Could you check a few things on this model? Use its own coordinates, in mm. A direction names the side the tool comes from. Coordinates: 2 decimals unless noted, no trailing zeros. Loops run counter-clockwise (first coordinate to the right, second up) from the corner with the lowest first, then second, coordinate; pieces in that order, holes last.
from build123d import *

# Parameters (mm, degrees)
BOSS_EXTRUDE1_DEPTH     = 18
CUT_EXTRUDE1_REACH      = 86.238
CUT_EXTRUDE1_END_RADIUS = 15
SKETCH3_R               = 7


with BuildPart() as part:
    # Sketch2 → Boss-Extrude1 (new body)
    with BuildSketch(Plane.XY):
        with BuildLine():
            Line((-33.38706816, 74), (-36, 74))
            Line((-36, 74), (-36, 0))
            Line((-36, 0), (-33, 0))
            Line((-33, 0), (-33, 35))
            ThreePointArc((-33, 35), (-18, 50), (-3, 35))
            Line((-3, 35), (-3, 0))
            Line((-3, 0), (0, 0))
            Line((0, 0), (0, 74))
            Line((0, 74), (-12.61679677, 74))
            Line((-12.61679677, 74), (-33.38706816, 74))
        make_face()
    extrude(amount=BOSS_EXTRUDE1_DEPTH)

    # Cut-Extrude1: up to this cylinder (the profile starts outside it)
    cut_extrude1_end = Plane(origin=(-18, 35, 9), z_dir=(0, 0, -1)) * Cylinder(CUT_EXTRUDE1_END_RADIUS, 203.476, mode=Mode.PRIVATE)
    # Sketch3 → Cut-Extrude1 (cut, up to the surface)
    with BuildSketch(Plane(origin=(0, 74, 0), x_dir=(1, 0, 0), z_dir=(0, 1, 0)), mode=Mode.PRIVATE) as cut_extrude1_sk1:
        with Locations(Location((-18, -9, 0), (0, 0, 270))):
            Circle(SKETCH3_R)
    cut_extrude1_tool1 = extrude(cut_extrude1_sk1.sketch, amount=-CUT_EXTRUDE1_REACH, mode=Mode.PRIVATE) - cut_extrude1_end
    add(cut_extrude1_tool1.solids().sort_by_distance((-18, 74, 9))[0], mode=Mode.SUBTRACT)


solid = part.part
(1) Imagine slicing it at D-D, the plane y = 67. Write out the boundary of the cut face in (x, z), and give its area (3 significant figures).
Answers:
outline: (-36, 0) - (0, 0) - (0, 18) - (-36, 18) - close; hole circle Ø14 at (-18, 9)
area: 494 mm2
(2) Imagine slicing it at A-A, the plane y = 8. Write out the boundary of the cut face in (x, z), and give its area (3 significant figures).
Answers:
outline: (-36, 0) - (-33, 0) - (-33, 18) - (-36, 18) - close; (-3, 0) - (0, 0) - (0, 18) - (-3, 18) - close
area: 108 mm2
(3) Which directions (+Z, -Z, +X, -X, +Y, -Y) give clear straight access to the entire face, cutting with the end or side of a thin tool? Please do faces 1 (the face through (-2, 0, 9)), 2 (the face through (-33, 17, 9)).
Answers:
face 1: +Z, -Z, +X, -X, -Y
face 2: +Z, -Z, -Y
(4) Imagine slicing it at B-B, the plane x = -18. Write out the boundary of the cut face in (y, z), and give its area (3 significant figures).
Answers:
outline: (50, 0) - (74, 0) - (74, 2) - (50, 2) - close; (50, 16) - (74, 16) - (74, 18) - (50, 18) - close
area: 96.0 mm2
(5) For pin 1 (6 mm diameter, centred on x = -4, z = 2.5, fed in from -Y); pin 2 (1.5 mm diameter, centred on x = -9.5, z = 2.5, fed in from -Y); pin 3 (8 mm diameter, centred on x = -10.5, y = 39.5, fed in from +Z), each with a flat end and sliding along its axis, tell me the tip position at first contact or that it passes through.
Answers:
pin 1: stops at y = 0
pin 2: stops at y = 46.81
pin 3: passes through
(6) We'd pull the mould along X, two halves only. Please class faces 3 (the face through (0, 36, 9)), 4 (the face through (-3, 18, 9)), 5 (the face through (-18, 54, 18)), 6 (the face through (-36, 38, 9)): +X half, -X half, draft (parallel to the pull), parting line (faces both ways), or undercut.
Answers:
face 3: +X half
face 4: undercut
face 5: draft
face 6: -X half
(7) I need wall thicknesses on probe 1 along X at (y, z) = (3, 8.25); probe 2 along X at (y, z) = (55.5, 9); probe 3 along Z at (x, y) = (-18, 54). Which ranges of each line are inside material? Lowest first, please.
Answers:
probe 1: x = -36 to -33, -3 to 0
probe 2: x = -36 to -25, -11 to 0
probe 3: z = 0 to 2, 16 to 18
(8) Imagine slicing it at C-C, the plane z = 14.5. Write out the boundary of the cut face in (x, y).
Answers:
outline: (-36, 0) - (-33, 0) - (-33, 35) arc R15 cw to (-22.33, 49.36) - (-22.33, 74) - (-36, 74) - close; (-13.67, 49.36) arc R15 cw to (-3, 35) - (-3, 0) - (0, 0) - (0, 74) - (-13.67, 74) - close
